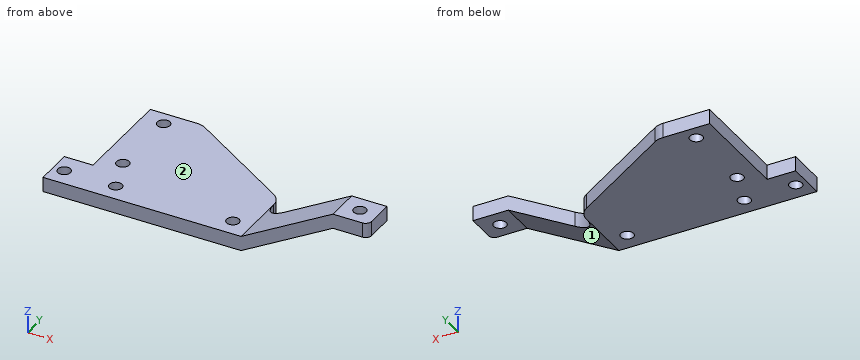
from build123d import *

# Parameters (mm, degrees)
SKETCH_R        = 4.3
PAD_DEPTH       = 10
PAD001_DEPTH    = 23
FILLET_R        = 17
SKETCH002_R     = 4.3
POCKET_DEPTH    = 45.001
FILLET001_R     = 4
SKETCH003_R     = 4.3
POCKET001_DEPTH = 10.001
CHAMFER_SIZE2   = 80
CHAMFER_SIZE    = 50
FILLET002_R     = 11.9


with BuildPart() as part:
    # Sketch → Pad (new body)
    with BuildSketch(Plane.XY):
        Polygon((0.4, 70), (0.4, -0.4), (-19, -0.4), (-19, -26.6), (115.6, -26.6), (115.6, 0), (115.6, 70), align=None)
        with Locations((15, 60)):
            Circle(SKETCH_R, mode=Mode.SUBTRACT)
        with Locations((15, 10)):
            Circle(SKETCH_R, mode=Mode.SUBTRACT)
    extrude(amount=PAD_DEPTH)

    # Sketch001 (on Face4 of Pad) → Pad001 (join)
    with BuildSketch(Plane.XZ.offset(26.6)):
        Polygon((115.6, 0), (178, 35), (202, 35), (202, 45), (178, 45), (115.6, 10), align=None)
    extrude(amount=-PAD001_DEPTH)

    # Fillet
    fillet_edges = [part.edges().sort_by_distance(p)[0] for p in [
        (115.6, -3.6, 5),
    ]]
    fillet(fillet_edges, radius=FILLET_R)

    # Sketch002 (on Face16 of Fillet) → Pocket (cut, through all)
    with BuildSketch(Plane.XY.offset(45)):
        with Locations((190, -15.1)):
            Circle(SKETCH002_R)
    extrude(amount=-POCKET_DEPTH, mode=Mode.SUBTRACT)

    # Fillet001
    fillet001_edges = [part.edges().sort_by_distance(p)[0] for p in [
        (202, -26.6, 40),
    ]]
    fillet(fillet001_edges, radius=FILLET001_R)

    # Sketch003 (on Face9 of Fillet001) → Pocket001 (cut, through all)
    with BuildSketch(Plane.XY.offset(10)):
        with Locations((-11.5, -14.1)):
            Circle(SKETCH003_R)
        with Locations((23.5, -14.1)):
            Circle(SKETCH003_R)
        with Locations((103.1, -14.1)):
            Circle(SKETCH003_R)
    extrude(amount=-POCKET001_DEPTH, mode=Mode.SUBTRACT)

    # Chamfer
    chamfer_edges = [part.edges().sort_by_distance(p)[0] for p in [
        (115.6, 70, 5),
    ]]
    chamfer_side = part.faces().sort_by_distance((115.6, 41.7, 5))[0]
    chamfer(chamfer_edges, length=CHAMFER_SIZE, length2=CHAMFER_SIZE2, reference=chamfer_side)

    # Fillet002
    fillet002_edges = [part.edges().sort_by_distance(p)[0] for p in [
        (115.6, 20, 5),
        (35.6, 70, 5),
    ]]
    fillet(fillet002_edges, radius=FILLET002_R)


solid = part.part
Part model, mm, in its own coordinate system. Face numbers are marked on the shaded views. A direction names the side the tool comes from. Coordinates: 2 decimals unless noted, no trailing zeros. Write each loop counter-clockwise with the first axis right and the second up, starting at its lowest first coordinate (ties: lowest second). Pieces come first, ordered by that corner, then holes. Notation, with made-up numbers: M 62,-3 L 87,-3 A10 ccw 87,11 Z; hole C -8.5,-28 d4. An arc over 180 degrees is marked long. Return JSON: item names as keys, results as strings.
1. Saw through at C-C, the plane x = 15. Write the cut outline in (y, z), then the cut area to 3 significant figures.
Determined:
{"outline": "M -26.6,0 L 5.7,0 L 5.7,10 L -26.6,10 Z; M 14.3,0 L 55.7,0 L 55.7,10 L 14.3,10 Z; M 64.3,0 L 70,0 L 70,10 L 64.3,10 Z", "area": "794 mm²"}
2. Saw through at B-B, the plane y = 60. Write the cut outline in (x, z), then the cut area to 3 significant figures.
Determined:
{"outline": "M 0.4,0 L 10.7,0 L 10.7,10 L 0.4,10 Z; M 19.3,0 L 51.6,0 L 51.6,10 L 19.3,10 Z", "area": "426 mm²"}
3. Probe L1, parallel to Y at x = 15, z = 3; L2, parallel to Y at x = 103.1, z = 7; L3, parallel to Z at x = 61, y = 41. List the from-to ranges inside material, lowest first.
Determined:
{"L1": "-26.6 to 5.7, 14.3 to 55.7, 64.3 to 70", "L2": "-26.6 to -18.4, -9.8 to 27.81", "L3": "0 to 10"}
4. Flat gauge pins, fed straight in: pin 1 Ø11 at (x, y) = (23.5, -14.1) entering from +Z; pin 2 Ø5 at (y, z) = (31, 5.5) entering from -X; pin 3 Ø12 at (x, y) = (21, 25) entering from -Z; pin 4 Ø3 at (x, z) = (-6.5, 4.5) entering from +Y. Where does each tip first touch, or does it go through?
Determined:
{"pin 1": "z = 10", "pin 2": "x = 0.4", "pin 3": "z = 0", "pin 4": "y = -0.4"}
5. 3-axis set-ups, long thin cutter, end or side, ignore diameter. For the marked faces 1 and 2: which of +Z, -Z, +X, -X, +Y, -Y reach the whole face in a straight line?
Determined:
{"face 1": "-Z, +X, +Y, -Y", "face 2": "+Z, -X, +Y, -Y"}
6. Saw through at D-D, the plane z = 5. Count the separate pieces of the cut face and the enclosed holes in it, then the cut area to 3 significant figures.
Determined:
{"separate pieces": "1", "enclosed holes": "5", "area": "9,600 mm²"}
7. Saw through at A-A, the plane x = 190. Write the cut outline in (y, z), then the cut area to 3 significant figures.
Determined:
{"outline": "M -26.6,35 L -19.4,35 L -19.4,45 L -26.6,45 Z; M -10.8,35 L -3.6,35 L -3.6,45 L -10.8,45 Z", "area": "144 mm²"}
